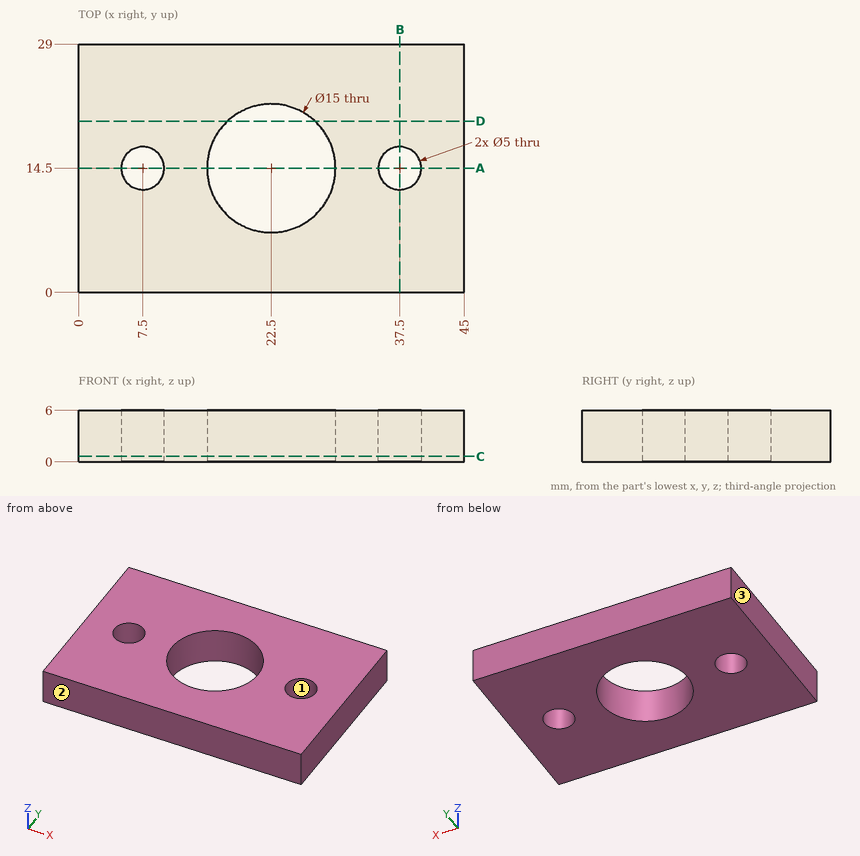
Drawing for the job (mm, zero at the part's lowest x, y, z). Give positions to 0.01 mm unless a question says otherwise; leave off trailing zeros. Order: outer loops, then holes, each group sorted by start corner. A loop starts at its lowest first (then second) coordinate and runs counter-clockwise, first axis right, second up. Notation, with made-up numbers: M 81.25,16 L 97.25,16 A6 ccw 97.25,22 Z; hole C 54,-12.5 d11. An arc over 180 degrees is marked long. Write item = value, one per line. Start each with the question number.
(1) Slice it at B-B on x = 37.5. Write the cut outline in (y, z).
(2) Slice it at A-A on y = 14.5. Write the cut outline in (x, z).
(3) Two-plate mould, pull along X, no slides. Class the marked faces 1, 2 and 3: released by +X, released by -X, zero draft, split by the parting line, or undercut.
(4) Slice it at D-D on y = 20. Write the cut outline in (x, z).
(5) Probe L1, parallel to X at y = 15, z = 1.9; L2, parallel to Y at x = 22.5, z = 2.85; L3, parallel to Y at x = 37.5, z = 3.75. List the from-to ranges inside material, lowest first. Write a range as [from, to].
(6) Slice it at C-C on z = 0.65. Write the cut outline in (x, y).
Responses:
q1.outline = M 0,0 L 12,0 L 12,6 L 0,6 Z; M 17,0 L 29,0 L 29,6 L 17,6 Z
q2.outline = M 0,0 L 5,0 L 5,6 L 0,6 Z; M 10,0 L 15,0 L 15,6 L 10,6 Z; M 30,0 L 35,0 L 35,6 L 30,6 Z; M 40,0 L 45,0 L 45,6 L 40,6 Z
q3.face_1 = undercut
q3.face_2 = zero draft
q3.face_3 = released by -X
q4.outline = M 0,0 L 17.4,0 L 17.4,6 L 0,6 Z; M 27.6,0 L 45,0 L 45,6 L 27.6,6 Z
q5.L1 = [0, 5.05], [9.95, 15.02], [29.98, 35.05], [39.95, 45]
q5.L2 = [0, 7], [22, 29]
q5.L3 = [0, 12], [17, 29]
q6.outline = M 0,0 L 45,0 L 45,29 L 0,29 Z; hole C 7.5,14.5 d5; hole C 22.5,14.5 d15; hole C 37.5,14.5 d5
